from build123d import *

# Parameters (mm, degrees)
SKETCH1_W           = 63.5
SKETCH1_H           = 101.6
BOSS_EXTRUDE1_DEPTH = 50.8
SHELL1_T            = -2.54
SKETCH2_W           = 6.35
SKETCH2_H           = 101.6
BOSS_EXTRUDE2_DEPTH = 4.572


with BuildPart() as part:
    # Sketch1 → Boss-Extrude1 (new body)
    with BuildSketch(Plane(origin=(0, 0, 0), x_dir=(1, 0, 0), z_dir=(0, 1, 0))):
        with Locations((31.75, 50.8)):
            Rectangle(SKETCH1_W, SKETCH1_H)
    extrude(amount=BOSS_EXTRUDE1_DEPTH)

    # Shell1
    shell1_openings = [part.faces().sort_by_distance(p)[0] for p in [
        (31.75, 50.8, -50.8),
    ]]
    offset(amount=SHELL1_T, openings=shell1_openings, kind=Kind.INTERSECTION)

    # Sketch2 → Boss-Extrude2 (add)
    with BuildSketch(Plane(origin=(0, 50.8, 0), x_dir=(1, 0, 0), z_dir=(0, 1, 0))):
        with Locations((-3.175, 50.8)):
            Rectangle(SKETCH2_W, SKETCH2_H)
        with Locations((66.675, 50.8)):
            Rectangle(SKETCH2_W, SKETCH2_H)
    extrude(amount=-BOSS_EXTRUDE2_DEPTH)


solid = part.part
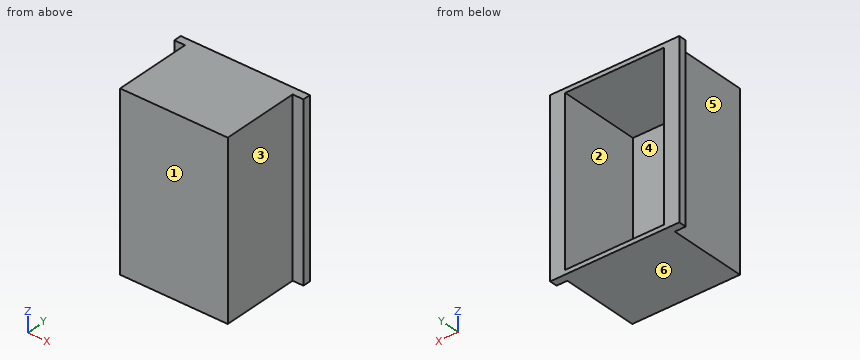
CAD build for the part. Positions are in the model's coordinates, mm. Face numbers are marked on the shaded views. A direction names the side the tool comes from. Give positions to 0.01 mm unless a question says otherwise; leave off trailing zeros. Loops run counter-clockwise (first coordinate to the right, second up) from the corner with the lowest first, then second, coordinate; pieces in that order, holes last. Notation, with made-up numbers: M 72.25,64 L 107.25,64 A35 cw 107.25,99 Z; hole C 43.5,48 d9. An arc over 180 degrees is marked long. Answer in a Markdown table with one row per item. Add a question column.
Item 1: Drop flat-ended pins along their axis: P1, Ø6, axis at y = 21.5, z = -65, coming from the -X side; P2, Ø5, axis at x = 44, z = -23, coming from the +Y side; P3, Ø14, axis at y = 23, z = -47.5, coming from the +X side. Give the stop position or say it passes through.
Item 2: Band-saw the part on C-C on z = -66. Give the cut face in (x, y).
Item 3: Band-saw the part on A-A on y = 45. Give the cut face in (x, z), then the cut area to 3 significant figures.
Item 4: Tool access for the marked faces 1 and 2: list every direction of +Z, -Z, +X, -X, +Y, -Y with a clear straight run to the whole face (end or side of a thin tool).
Item 5: Mould opens along X. For the marked faces 3, 4, 5 and 6 say: +X half, -X half, draft (parallel to the pull), parting line (faces both ways), or undercut.
Item 6: Band-saw the part on B-B on x = 55. Give the cut face in (y, z).
Item 7: Probe probe 1 along Z at (x, y) = (29, 15); probe 2 along X at (y, z) = (24, -42.5); probe 3 along Y at (x, z) = (16, -38). List the from-to ranges inside material, lowest first.
Reply:
| question | item | result |
|---|---|---|
| 1 | P1 | stops at x = 0 |
| 1 | P2 | stops at y = 2.54 |
| 1 | P3 | stops at x = 63.5 |
| 2 | outline | M -6.35,46.23 L 0,46.23 L 0,0 L 63.5,0 L 63.5,46.23 L 69.85,46.23 L 69.85,50.8 L 60.96,50.8 L 60.96,2.54 L 2.54,2.54 L 2.54,50.8 L -6.35,50.8 Z |
| 3 | outline | M 0,-101.6 L 63.5,-101.6 L 63.5,0 L 0,0 Z; hole M 2.54,-99.06 L 60.96,-99.06 L 60.96,-2.54 L 2.54,-2.54 Z |
| 3 | area | 813 mm^2 |
| 4 | face 1 | +Z, -Z, +X, -X, -Y |
| 4 | face 2 | +Y |
| 5 | face 3 | +X half |
| 5 | face 4 | undercut |
| 5 | face 5 | -X half |
| 5 | face 6 | draft |
| 6 | outline | M 0,-101.6 L 50.8,-101.6 L 50.8,-99.06 L 2.54,-99.06 L 2.54,-2.54 L 50.8,-2.54 L 50.8,0 L 0,0 Z |
| 7 | probe 1 | z = -101.6 to -99.06, -2.54 to 0 |
| 7 | probe 2 | x = 0 to 2.54, 60.96 to 63.5 |
| 7 | probe 3 | y = 0 to 2.54 |
